```python
from build123d import *

# Parameters (mm, degrees)
F0_W     = 165
F0_H     = 30
F0_R     = 1.5
F0_R_2   = 4.75
F0_R_3   = 2.055
F1_DEPTH = 10
F2_DEPTH = 2.75
F3_DEPTH = 25


with BuildPart() as f1:
    # F0 (on Front) → F1 (new body)
    with BuildSketch(Plane.XZ):
        Rectangle(F0_W, F0_H)
        with Locations((-77.5, 0)):
            Circle(F0_R, mode=Mode.SUBTRACT)
        Circle(F0_R_2, mode=Mode.SUBTRACT)
        with Locations((77.5, 0)):
            Circle(F0_R, mode=Mode.SUBTRACT)
        Circle(F0_R_2)
        Circle(F0_R_3, mode=Mode.SUBTRACT)
        Circle(F0_R_3)
    extrude(amount=F1_DEPTH)

    # F0 (on Front) → F2 (cut)
    with BuildSketch(Plane.XZ):
        Circle(F0_R_2)
        Circle(F0_R_3, mode=Mode.SUBTRACT)
        Circle(F0_R_3)
    extrude(amount=F2_DEPTH, mode=Mode.SUBTRACT)

    # F0 (on Front) → F3 (cut)
    with BuildSketch(Plane.XZ):
        Circle(F0_R_3)
    extrude(amount=F3_DEPTH, mode=Mode.SUBTRACT)


solid = f1.part
```
Geometry: final body of the model. Coordinates: model frame, mm. A direction names the side the tool comes from. Coordinates: 2 decimals unless noted, no trailing zeros. Write each loop counter-clockwise with the first axis right and the second up, starting at its lowest first coordinate (ties: lowest second). Pieces come first, ordered by that corner, then holes. Notation, with made-up numbers: M 76,83.25 L 92,83.25 A24 cw 92,108.25 Z; hole C 31,43.25 d5. An arc over 180 degrees is marked long. Use CSV: the item, a comma, the result in double quotes. Start each with the question number.
1. Cut plane A-A on x = 0. Return the cut outline in (y, z) (3 decimals), plus the area to 3 significant figures.
2. Ray query, probe 1 along X at (y, z) = (-4.75, -0.5); probe 2 along Z at (x, y) = (0, -0.8); probe 3 along Z at (x, y) = (0, -6) (3 decimals). Return the intervals inside material, ascending.
3. First-contact query: P1, Ø6.5, axis at x = 0, z = 0, coming from the +Y side. Flat tip, straight axial feed; report the tip coordinate or a pass-through.
4. Reachability of faces 4 (the face through (-0.445, -6.324, -2.006)), 5 (the face through (2, -2.75, -1)) from +Z, -Z, +X, -X, +Y, -Y: full face, straight path, thin tool, end or side. Return the list, or none.
5. Cut plane C-C on x = -77.5. Return the cut outline in (y, z), plus the area to 3 significant figures.
6. Cut plane B-B on z = 0. Return the cut outline in (x, y) (3 decimals), plus the area to 3 significant figures.
7. Mould query, pull axis X, two halves, no side actions, for faces 1 (the face through (-82.5, -5, 0)), 2 (the face through (79, -5, 0)), 3 (the face through (-1, -10, 4)). Classes: pulls with the +X half, pulls with the -X half, needs draft (parallel to the pull), parting line crosses it, or undercut.
Entries:
1,outline,"M -10,-15 L 0,-15 L 0,-4.75 L -2.75,-4.75 L -2.75,-2.055 L -10,-2.055 Z; M -10,2.055 L -2.75,2.055 L -2.75,4.75 L 0,4.75 L 0,15 L -10,15 Z"
1,area,"244 mm²"
2,probe 1,"-82.5 to -78.91, -76.09 to -1.99, 1.99 to 76.09, 78.91 to 82.5"
2,probe 2,"-15 to -4.75, 4.75 to 15"
2,probe 3,"-15 to -2.055, 2.055 to 15"
3,P1,"y = -2.75"
4,face 4,"+Y, -Y"
4,face 5,"+Y"
5,outline,"M -10,-15 L 0,-15 L 0,-1.5 L -10,-1.5 Z; M -10,1.5 L 0,1.5 L 0,15 L -10,15 Z"
5,area,"270 mm²"
6,outline,"M -82.5,-10 L -79,-10 L -79,0 L -82.5,0 Z; M -76,-10 L -2.055,-10 L -2.055,-2.75 L -4.75,-2.75 L -4.75,0 L -76,0 Z; M 2.055,-10 L 76,-10 L 76,0 L 4.75,0 L 4.75,-2.75 L 2.055,-2.75 Z; M 79,-10 L 82.5,-10 L 82.5,0 L 79,0 Z"
6,area,"1,530 mm²"
7,face 1,"pulls with the -X half"
7,face 2,"undercut"
7,face 3,"needs draft"
